Could you check a few things on this model? Use its own coordinates, in mm. A direction names the side the tool comes from. Coordinates: 2 decimals unless noted, no trailing zeros. Write each loop counter-clockwise with the first axis right and the second up, starting at its lowest first coordinate (ties: lowest second). Pieces come first, ordered by that corner, then holes.
```python
from build123d import *

# Parameters (mm, degrees)
SKETCH005_R   = 2
SKETCH005_R_2 = 2.65
PAD_DEPTH     = 4
FILLET_R      = 5
FILLET001_R   = 1
FILLET002_R   = 1


with BuildPart() as part:
    # Sketch005 → Pad (new body)
    with BuildSketch(Plane.XY.offset(-3)):
        Polygon((-38, 10), (-31, 10), (-31, 1), (-37, 1), (-37, -1), (-31, -1), (-31, -10), (9, -10), (9, -1), (15, -1), (15, 1), (9, 1), (9, 10), (17, 10), (47, 0.7), (47, -8.030345), (28, -19), (-35, -19), (-50, -10.339746), (-50, 3.07), align=None)
        with Locations((-35.5, 5)):
            Circle(SKETCH005_R, mode=Mode.SUBTRACT)
        with Locations((-35.5, -5)):
            Circle(SKETCH005_R, mode=Mode.SUBTRACT)
        with Locations((13.5, 5)):
            Circle(SKETCH005_R, mode=Mode.SUBTRACT)
        with Locations((13.5, -5)):
            Circle(SKETCH005_R, mode=Mode.SUBTRACT)
        with Locations((-44.5, 0)):
            Circle(SKETCH005_R_2, mode=Mode.SUBTRACT)
        with Locations((40.5, -5)):
            Circle(SKETCH005_R_2, mode=Mode.SUBTRACT)
    extrude(amount=PAD_DEPTH)

    # Fillet
    fillet_edges = [part.edges().sort_by_distance(p)[0] for p in [
        (28, -19, -1),
        (47, -8.030345, -1),
        (-35, -19, -1),
        (-50, -10.339746, -1),
        (-50, 3.07, -1),
        (-38, 10, -1),
        (47, 0.7, -1),
        (17, 10, -1),
        (-31, 10, -1),
        (9, 10, -1),
    ]]
    fillet(fillet_edges, radius=FILLET_R)

    # Fillet001
    fillet001_edges = [part.edges().sort_by_distance(p)[0] for p in [
        (-31, -10, -1),
        (9, -10, -1),
    ]]
    fillet(fillet001_edges, radius=FILLET001_R)

    # Fillet002
    fillet002_edges = [part.edges().sort_by_distance(p)[0] for p in [
        (-31, -1, -1),
        (-31, 1, -1),
        (9, 1, -1),
        (9, -1, -1),
    ]]
    fillet(fillet002_edges, radius=FILLET002_R)


solid = part.part
```
Item 1: I want a section at B-B, the plane x = 40.5. List the corners of the cut face in (y, z) for me (3 decimals).
Item 2: If I drill on line 1 along Y through (x, z) = (13.5, -0.15); line 2 along Y through (x, z) = (-35.5, -1.6); line 3 along Y through (x, z) = (-28.5, -0.2), over which ranges is the centre line in solid material (lowest first)?
Item 3: Which directions (+Z, -Z, +X, -X, +Y, -Y) give clear straight access to the entire face, cutting with the end or side of a thin tool? Please do faces 1 (the flat face through (-35, -1, -1)), 2 (the cylindrical face through (46.31, -7.68, -0.97)), 3 (the flat face through (-11, -10, -1)).
Item 4: I want a section at A-A, the plane y = 8. List the corners of the cut face in (x, z) for me.
Item 5: Will these pins go through, and if not, where does the flat tip stop? pin 1 Ø3 at (x, y) = (-35.5, -5) entering from +Z; pin 2 Ø2 at (y, z) = (-10.5, -1) entering from +X; pin 3 Ø2 at (x, z) = (-34.5, -1.5) entering from -Y; pin 4 Ø0.6 at (y, z) = (0.5, -1) entering from +X.
Item 6: I want a section at D-D, the plane x = -24.5. List the corners of the cut face in (y, z) for me, then the cut area to 3 significant figures.
Item 7: I want a section at C-C, the plane z = -0.15. Count the separate pieces of the cut face and the enclosed holes in it, then the cut area to 3 significant figures.
Taken from the geometry:
1. outline: (-11.783, -3) - (-7.65, -3) - (-7.65, 1) - (-11.783, 1) - close; (-2.35, -3) - (2.715, -3) - (2.715, 1) - (-2.35, 1) - close
2. line 1: y = -19 to -7, -3 to -1, 1 to 3, 7 to 9.97
2. line 2: y = -18.65 to -7, -3 to -1, 1 to 3, 7 to 9.97
2. line 3: y = -19 to -10
3. face 1: +Z, -Z
3. face 2: +Z, -Z, +X, -Y
3. face 3: +Z, -Z, +Y
4. outline: (-41.46, -3) - (-32, -3) - (-32, 1) - (-41.46, 1) - close; (10, -3) - (23.45, -3) - (23.45, 1) - (10, 1) - close
5. pin 1: passes through
5. pin 2: stops at x = 44.45
5. pin 3: stops at y = -19
5. pin 4: stops at x = 45.85
6. outline: (-19, -3) - (-10, -3) - (-10, 1) - (-19, 1) - close
6. area: 36.0 mm2
7. separate pieces: 1
7. enclosed holes: 6
7. area: 1,530 mm2
